```python
from build123d import *

# Parameters (mm, degrees)
SKETCH_1_R           = 27.5
SKETCH_1_R_2         = 6.6
SKETCH_1_R_3         = 1.3
EXTRUDE_1_DEPTH      = 7
SKETCH_2_R           = 2.5
CUT_EXTRUDE_2_DEPTH  = 5
SKETCH_4_R           = 1
CUT_EXTRUDE_3_DEPTH  = 6
SKETCH_5_R           = 1.5
CUT_EXTRUDE_4_DEPTH  = 50.019507543
CUT_EXTRUDE_5_DEPTH  = 2.7
CUT_EXTRUDE_6_DEPTH  = 10
FILLET_1_R           = 1
SKETCH_9_R           = 2.1
EXTRUDE_3_DEPTH      = 7
SKETCH_13_R          = 1
CUT_EXTRUDE_9_DEPTH  = 88.1614895
SKETCH_14_R          = 2.1
EXTRUDE_4_DEPTH      = 22
FILLET_2_R           = 16
SKETCH_15_R          = 1.5
CUT_EXTRUDE_10_DEPTH = 91.308323515
SKETCH_16_R          = 3
CUT_EXTRUDE_11_DEPTH = 3
SKETCH_17_R          = 5


with BuildPart() as part:
    # 草图1 → 凸台-拉伸1 (new body)
    with BuildSketch(Plane(origin=(0, 0, 0), x_dir=(1, 0, 0), z_dir=(0, 1, 0))):
        with Locations(Location((0, -12.470765814, 0), (0, 0, 270))):
            Circle(SKETCH_1_R)
        with Locations(Location((0, -12.470765814, 0), (0, 0, 270))):
            Circle(SKETCH_1_R_2, mode=Mode.SUBTRACT)
        with Locations(Location((-10.8, -18.706148722, 0), (0, 0, 270))):
            Circle(SKETCH_1_R_3, mode=Mode.SUBTRACT)
        with Locations(Location((10.8, -18.706148722, 0), (0, 0, 270))):
            Circle(SKETCH_1_R_3, mode=Mode.SUBTRACT)
        with Locations(Location((0, 0, 0), (0, 0, 270))):
            Circle(SKETCH_1_R_3, mode=Mode.SUBTRACT)
    extrude(amount=EXTRUDE_1_DEPTH)

    # 草图2 → 切除-拉伸2 (cut)
    with BuildSketch(Plane(origin=(0, 7, 0), x_dir=(1, 0, 0), z_dir=(0, 1, 0))):
        with Locations(Location((-10.8, -18.706148722, 0), (0, 0, 270))):
            Circle(SKETCH_2_R)
        with Locations(Location((10.8, -18.706148722, 0), (0, 0, 270))):
            Circle(SKETCH_2_R)
        with Locations(Location((0, 0, 0), (0, 0, 270))):
            Circle(SKETCH_2_R)
    extrude(amount=-CUT_EXTRUDE_2_DEPTH, mode=Mode.SUBTRACT)

    # 草图4 → 切除-拉伸3 (cut)
    with BuildSketch(Plane(origin=(0, 7, 0), x_dir=(1, 0, 0), z_dir=(0, 1, 0))):
        with Locations(Location((-6.92820323, -8.470765814, 0), (0, 0, 270))):
            Circle(SKETCH_4_R)
        with Locations(Location((6.92820323, -8.470765814, 0), (0, 0, 90))):
            Circle(SKETCH_4_R)
        with Locations(Location((0, -20.470765814, 0), (0, 0, 270))):
            Circle(SKETCH_4_R)
    extrude(amount=-CUT_EXTRUDE_3_DEPTH, mode=Mode.SUBTRACT)

    # 草图5 → 切除-拉伸4 (cut, through all)
    with BuildSketch(Plane(origin=(0, 7, 0), x_dir=(1, 0, 0), z_dir=(0, 1, 0))):
        with Locations(Location((-17.320508076, -2.470765814, 0), (0, 0, 270))):
            Circle(SKETCH_5_R)
        with Locations(Location((0, -32.470765814, 0), (0, 0, 270))):
            Circle(SKETCH_5_R)
        with Locations(Location((17.320508076, -2.470765814, 0), (0, 0, 270))):
            Circle(SKETCH_5_R)
    extrude(amount=-CUT_EXTRUDE_4_DEPTH, mode=Mode.SUBTRACT)

    # 草图6 → 切除-拉伸5 (cut)
    with BuildSketch(Plane.XZ):
        Polygon((3.290896534, 32.470765814), (1.645448267, 35.320765814), (-1.645448267, 35.320765814), (-3.290896534, 32.470765814), (-1.645448267, 29.620765814), (1.645448267, 29.620765814), align=None)
        Polygon((20.61140461, 2.470765814), (18.965956343, 5.320765814), (15.675059808, 5.320765814), (14.029611541, 2.470765814), (15.675059808, -0.379234186), (18.965956343, -0.379234186), align=None)
        Polygon((-14.029611541, 2.470765814), (-15.675059808, 5.320765814), (-18.965956343, 5.320765814), (-20.61140461, 2.470765814), (-18.965956343, -0.379234186), (-15.675059808, -0.379234186), align=None)
    extrude(amount=-CUT_EXTRUDE_5_DEPTH, mode=Mode.SUBTRACT)

    # 草图7 → 切除-拉伸6 (cut)
    with BuildSketch(Plane(origin=(0, 7, 0), x_dir=(1, 0, 0), z_dir=(0, 1, 0))):
        Polygon((19.338457268, -14.975575286), (11.838457268, -27.965956343), (14.003520778, -29.215956343), (21.468764488, -16.285774946), align=None)
    extrude(amount=-CUT_EXTRUDE_6_DEPTH, mode=Mode.SUBTRACT)

    # 圆角1
    fillet_1_edges = [part.edges().sort_by_distance(p)[0] for p in [
        (15.588457268, 0, 21.470765814),
        (17.736142633, 0, 22.750865644),
        (15.588457268, 7, 21.470765814),
        (17.736142633, 7, 22.750865644),
    ]]
    fillet(fillet_1_edges, radius=FILLET_1_R)

    # 草图9 → 凸台-拉伸3 (add)
    with BuildSketch(Plane.XZ):
        with BuildLine():
            Line((-24.637772228, 24.686746318), (-70.563132874, -13.924926133))
            ThreePointArc((-70.563132874, -13.924926133), (-75.458515455, -31.192547657), (-58.048161541, -35.553178381))
            Line((-58.048161541, -35.553178381), (-1.686469289, -14.977473133))
            Line((-1.686469289, -14.977473133), (-0.82500702, -15.016856189))
            Line((-0.82500702, -15.016856189), (-16.980808265, -9.160280176))
            Line((-16.980808265, -9.160280176), (-27.376809202, 9.870704679))
            Line((-27.376809202, 9.870704679), (-24.198243857, 25.535795253))
            Line((-24.198243857, 25.535795253), (-24.637772228, 24.686746318))
        make_face()
        with Locations(Location((-64.305647208, -24.739052257, 0), (0, 0, 270))):
            Circle(SKETCH_9_R, mode=Mode.SUBTRACT)
        Polygon((-58.808031517, -25.255019032), (-51.450927664, -20.997904645), (-52.552769035, -19.09371306), (-59.909872887, -23.350827447), align=None, mode=Mode.SUBTRACT)
    extrude(amount=-EXTRUDE_3_DEPTH)

    # 草图13 → 切除-拉伸9 (cut, through all)
    with BuildSketch(Plane(origin=(0, 7, 0), x_dir=(1, 0, 0), z_dir=(0, 1, 0))):
        with Locations(Location((4.029784687, -35.157765041, 0), (0, 0, 270))):
            Circle(SKETCH_13_R)
        with Locations(Location((21.824784687, -4.33592092, 0), (0, 0, 270))):
            Circle(SKETCH_13_R)
        with Locations(Location((-16.340954858, 17.69907908, 0), (0, 0, 270))):
            Circle(SKETCH_13_R)
        with Locations(Location((-34.135954858, -13.122765041, 0), (0, 0, 270))):
            Circle(SKETCH_13_R)
    extrude(amount=-CUT_EXTRUDE_9_DEPTH, mode=Mode.SUBTRACT)

    # 草图14 → 凸台-拉伸4 (add)
    with BuildSketch(Plane(origin=(0, 7, 0), x_dir=(1, 0, 0), z_dir=(0, 1, 0))):
        with BuildLine():
            Line((-70.563132874, 13.924926133), (-54.154588064, 0.129468707))
            Line((-54.154588064, 0.129468707), (-32.28086935, 26.146430855))
            Line((-32.28086935, 26.146430855), (-58.048161541, 35.553178381))
            ThreePointArc((-58.048161541, 35.553178381), (-74.791319703, 30.806481525), (-70.563132874, 13.924926133))
        make_face()
        with Locations(Location((-64.305647208, 24.739052257, 0), (0, 0, 90))):
            Circle(SKETCH_14_R, mode=Mode.SUBTRACT)
        Polygon((-58.808031517, 25.255019032), (-59.909872887, 23.350827447), (-52.552769035, 19.09371306), (-51.450927664, 20.997904645), align=None, mode=Mode.SUBTRACT)
    extrude(amount=EXTRUDE_4_DEPTH)

    # 圆角2
    fillet_2_edges = [part.edges().sort_by_distance(p)[0] for p in [
        (-43.217728707, 7, -13.137949781),
    ]]
    fillet(fillet_2_edges, radius=FILLET_2_R)

    # 草图15 → 切除-拉伸10 (cut, through all)
    with BuildSketch(Plane(origin=(-3.803339533, 0, 6.572894544), x_dir=(0.8655416297077619, 0, 0.5008369866961021), z_dir=(-0.5008369866961021, 0, 0.865541629707762))):
        with Locations(Location((-54.416791824, 23.665181086, 0), (0, 0, 245.053604138))):
            Circle(SKETCH_15_R)
    extrude(amount=-CUT_EXTRUDE_10_DEPTH, mode=Mode.SUBTRACT)

    # 草图16 → 切除-拉伸11 (cut)
    with BuildSketch(Plane(origin=(4.626421242, 0, -12.672855056), x_dir=(-0.9393615375389992, 0, -0.3429284207999792), z_dir=(0.3429284207999792, 0, -0.9393615375389992))):
        with Locations((53.038314469, 23.665181086)):
            Circle(SKETCH_16_R)
    extrude(amount=-CUT_EXTRUDE_11_DEPTH, mode=Mode.SUBTRACT)

    # 草图17 → 切除-旋转1 (revolve, cut)
    with BuildSketch(Plane(origin=(-31.791422565, 0, -26.728586941), x_dir=(0.6435278741872098, 0, -0.7654226774430521), z_dir=(0.7654226774430521, 0, 0.6435278741872098)), mode=Mode.PRIVATE) as cut_revolve_1_sk:
        with Locations((-25.901195998, 17.59703733)):
            Circle(SKETCH_17_R)
    revolve(cut_revolve_1_sk.sketch.rotate(Axis((-59.195395552, 24.020808836, 5.866150937), (0, -1, 0)), 329.642648375), axis=Axis((-59.195395552, 24.020808836, 5.866150937), (0, -1, 0)), mode=Mode.SUBTRACT)


solid = part.part
```
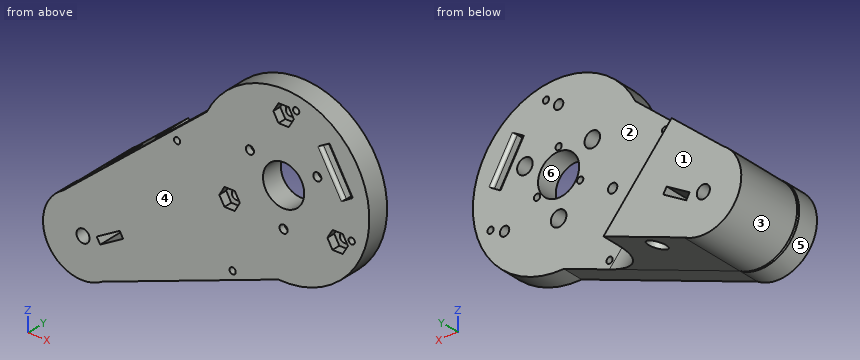
Design review of the part built by this model. Coordinates are the model's own, in mm. Face numbers are marked on the shaded views. A direction names the side the tool comes from. Coordinates: 2 decimals unless noted, no trailing zeros.
1) Mouldability with a two-part tool opening along X and no side actions: class the marked faces 4, 5 and 6 as +X half, -X half, draft (parallel to the pull), parting line (faces both ways), or undercut.
2) Wall thickness on line 1 along Z through (x, y) = (-63, 8); line 2 along Y through (x, z) = (-42.5, -8); line 3 along Y through (x, z) = (14.5, -6): over which ranges is each line inside the solid? List them lowest first.
3) For the marked faces 1, 2 and 3, list the 3-axis set-ups (+Z, -Z, +X, -X, +Y, -Y) from which the entire face can be reached by the end or side of a thin tool; tool diameter is ignored.
4) Take a section at A-A, the plane y = 4.5. State how many separate pieces and enclosed holes the cut face has, and give its area (3 significant figures).
5) Clearance check with flat-ended pins moving along their axes: pin 1 (3 mm diameter, centred on x = 21.82, z = 4.34, fed in from +Y); pin 2 (4 mm diameter, centred on x = 0, z = 32.47, fed in from -Y); pin 3 (15 mm diameter, centred on x = 0, z = 12.47, fed in from -Y); pin 4 (1.4 mm diameter, centred on x = -0.5, y = 1, fed in from -Z). State where each tip first meets the part, or that it passes through.
Returned:
1. face 4: draft
1. face 5: parting line
1. face 6: undercut
2. line 1: z = -37.01 to -26.38, -23.09 to -7.57
2. line 2: y = 0 to 12.58
2. line 3: y = 0 to 7
3. face 1: +Z, -Z, +X, -X, +Y
3. face 2: +Z, +X, +Y
3. face 3: +Y
4. separate pieces: 1
4. enclosed holes: 17
4. area: 4,020 mm2
5. pin 1: stops at y = 7
5. pin 2: stops at y = 2.7
5. pin 3: stops at y = 0
5. pin 4: stops at z = -15.03
